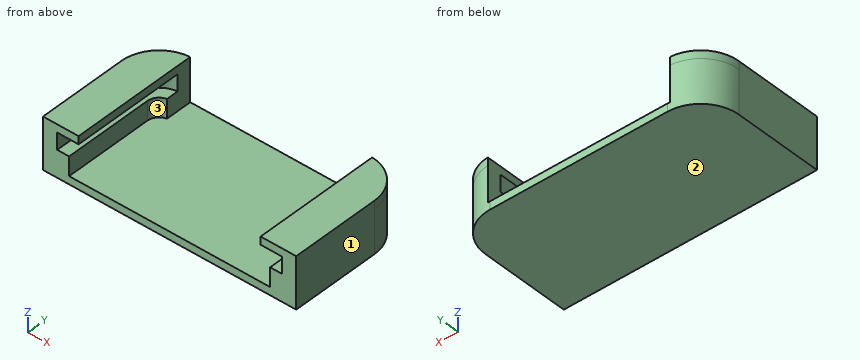
from build123d import *

# Parameters (mm, degrees)
BOSS_EXTRUDE2_DEPTH     = 5.5
CUT_EXTRUDE1_DEPTH      = 4.5
BOSS_EXTRUDE3_START     = 2.4
BOSS_EXTRUDE3_DEPTH     = 2.4
SALIENTE_EXTRUIR1_DEPTH = 1
CORTAR_EXTRUIR3_REACH   = 38.363
CROQUIS3_W              = 23
CROQUIS3_H              = 4.5


with BuildPart() as part:
    # Sketch3 → Boss-Extrude2 (new body)
    with BuildSketch(Plane.XY):
        with BuildLine():
            Line((0, 0), (32, 0))
            Line((32, 0), (32, 11.2))
            ThreePointArc((32, 11.2), (30.59411255, 14.59411255), (27.2, 16))
            Line((27.2, 16), (4.8, 16))
            ThreePointArc((4.8, 16), (1.40588745, 14.59411255), (0, 11.2))
            Line((0, 11.2), (0, 0))
        make_face()
    extrude(amount=BOSS_EXTRUDE2_DEPTH)

    # Sketch4 → Cut-Extrude1 (cut)
    with BuildSketch(Plane.XY.offset(5.5)):
        with BuildLine():
            Line((1.8, 0), (30.2, 0))
            Line((30.2, 0), (30.2, 11.2))
            ThreePointArc((30.2, 11.2), (29.321320344, 13.321320344), (27.2, 14.2))
            Line((27.2, 14.2), (4.8, 14.2))
            ThreePointArc((4.8, 14.2), (2.678679656, 13.321320344), (1.8, 11.2))
            Line((1.8, 11.2), (1.8, 0))
        make_face()
    extrude(amount=-CUT_EXTRUDE1_DEPTH, mode=Mode.SUBTRACT)

    # Sketch5 → Boss-Extrude3 (add)
    with BuildSketch(Plane.XY.offset(1).offset(BOSS_EXTRUDE3_START)):
        with BuildLine():
            Line((1.8, 11.2), (1.8, 0))
            Line((1.8, 0), (3.3, 0))
            Line((3.3, 0), (3.3, 11.2))
            ThreePointArc((3.3, 11.2), (3.739339828, 12.260660172), (4.8, 12.7))
            Line((4.8, 12.7), (27.2, 12.7))
            ThreePointArc((27.2, 12.7), (28.260660172, 12.260660172), (28.7, 11.2))
            Line((28.7, 11.2), (28.7, 0))
            Line((28.7, 0), (30.2, 0))
            Line((30.2, 0), (30.2, 11.2))
            ThreePointArc((30.2, 11.2), (29.321320344, 13.321320344), (27.2, 14.2))
            Line((27.2, 14.2), (4.8, 14.2))
            ThreePointArc((4.8, 14.2), (2.678679656, 13.321320344), (1.8, 11.2))
        make_face()
    extrude(amount=-BOSS_EXTRUDE3_DEPTH)

    # Croquis1 → Saliente-Extruir1 (add)
    with BuildSketch(Plane.XY.offset(5.5)):
        with BuildLine():
            Line((4.5, 0), (4.5, 15.990615827))
            ThreePointArc((4.5, 15.990615827), (1.301428863, 14.486335345), (0, 11.2))
            Line((0, 11.2), (0, 0))
            Line((0, 0), (4.5, 0))
        make_face()
        with BuildLine():
            Line((27.5, 15.990615827), (27.5, 0))
            Line((27.5, 0), (32, 0))
            Line((32, 0), (32, 11.2))
            ThreePointArc((32, 11.2), (30.698571137, 14.486335345), (27.5, 15.990615827))
        make_face()
    extrude(amount=SALIENTE_EXTRUIR1_DEPTH)

    # Croquis3 → Cortar-Extruir3 (cut, up to next)
    with BuildSketch(Plane(origin=(0, 16, 0), x_dir=(1, 0, 0), z_dir=(0, 1, 0)), mode=Mode.PRIVATE) as cortar_extruir3_sk1:
        with Locations((16, -3.25)):
            Rectangle(CROQUIS3_W, CROQUIS3_H)
    cortar_extruir3_tool1 = extrude(cortar_extruir3_sk1.sketch, amount=-CORTAR_EXTRUIR3_REACH, mode=Mode.PRIVATE) & part.part
    add(cortar_extruir3_tool1.solids().sort_by_distance((16, 16, 3.25))[0], mode=Mode.SUBTRACT)


solid = part.part
Build history of the part. All positions in model axes, mm. Face numbers are marked on the shaded views. Round coordinates to 2 decimals unless told otherwise and drop trailing zeros. Loops run counter-clockwise (first coordinate to the right, second up) from the corner with the lowest first, then second, coordinate; pieces in that order, holes last. Notation, with made-up numbers: (83, 15) -> (112, 15) arc R19 cw to (112, 30) -> close; hole circle Ø7 at (-26, 16). An arc over 180 degrees is marked (long way). Answer in a Markdown table with one row per item.
Item 1: Drill centre lines: L1, parallel to X at y = 3.5, z = 4; L2, parallel to X at y = 0.75, z = 6; L3, parallel to Z at x = 4, y = 1. Where is each one in solid material? Low to high. Write a range as [from, to].
Answers below:
| item | result |
|---|---|
| L1 | x = [0, 1.8], [30.2, 32] |
| L2 | x = [0, 4.5], [27.5, 32] |
| L3 | z = [0, 1], [5.5, 6.5] |
Item 2: Saw through at C-C (z = 2.75). Write the cut outline in (x, y).
Answers below:
| item | result |
|---|---|
| outline | (0, 0) -> (3.3, 0) -> (3.3, 11.2) arc R1.5 cw to (4.5, 12.67) -> (4.5, 15.99) arc R4.8 ccw to (0, 11.2) -> close; (27.5, 12.67) arc R1.5 cw to (28.7, 11.2) -> (28.7, 0) -> (32, 0) -> (32, 11.2) arc R4.8 ccw to (27.5, 15.99) -> close |
Item 3: Saw through at B-B (y = 10). Write the cut outline in (x, z).
Answers below:
| item | result |
|---|---|
| outline | (0, 0) -> (32, 0) -> (32, 6.5) -> (27.5, 6.5) -> (27.5, 5.5) -> (30.2, 5.5) -> (30.2, 3.4) -> (28.7, 3.4) -> (28.7, 1) -> (3.3, 1) -> (3.3, 3.4) -> (1.8, 3.4) -> (1.8, 5.5) -> (4.5, 5.5) -> (4.5, 6.5) -> (0, 6.5) -> close |
Item 4: Mould opens along Z. For the marked faces 1, 2 and 3 say: +Z half, -Z half, draft (parallel to the pull), parting line (faces both ways), or undercut.
Answers below:
| item | result |
|---|---|
| face 1 | draft |
| face 2 | -Z half |
| face 3 | undercut |
Item 5: Saw through at A-A (z = 4.25). Write the cut outline in (x, y).
Answers below:
| item | result |
|---|---|
| outline | (0, 0) -> (1.8, 0) -> (1.8, 11.2) arc R3 cw to (4.5, 14.18) -> (4.5, 15.99) arc R4.8 ccw to (0, 11.2) -> close; (27.5, 14.18) arc R3 cw to (30.2, 11.2) -> (30.2, 0) -> (32, 0) -> (32, 11.2) arc R4.8 ccw to (27.5, 15.99) -> close |
Item 6: Pin check, flat tips, straight feed: pin 1 (8 mm diameter, centred on x = 22.5, y = 9.5, fed in from +Z); pin 2 (1.5 mm diameter, centred on x = 26.5, z = 3.5, fed in from -Y). Stop position of each tip, or through.
Answers below:
| item | result |
|---|---|
| pin 1 | stops at z = 1 |
| pin 2 | passes through |
Item 7: Saw through at D-D (x = 4). Write the cut outline in (y, z), and give its area (3 significant figures).
Answers below:
| item | result |
|---|---|
| outline | (0, 0) -> (15.93, 0) -> (15.93, 6.5) -> (0, 6.5) -> (0, 5.5) -> (14.09, 5.5) -> (14.09, 3.4) -> (12.47, 3.4) -> (12.47, 1) -> (0, 1) -> close |
| area | 44.0 mm² |
